The model under review builds one solid part; all positions refer to its coordinate system, in mm. A direction names the side the tool comes from. Round coordinates to 2 decimals unless told otherwise and drop trailing zeros.
1) Consider section A-A (z = 4.5). Give the number of separate pieces and of enclosed holes in the cut face, then the cut area to 3 significant figures.
2) Machinability: for faces 4 (the face through (11.156, 1.113, 11.154)), 5 (the face through (0, 5, 11)), which of the approach directions +Z, -Z, +X, -X, +Y, -Y give a long, thin tool a straight path to every point of the face, cutting with its end or side? Answer none if there is none.
3) Clearance check with flat-ended pins moving along their axes: P1, Ø2, axis at x = 8, z = 4, coming from the +Y side; P2, Ø5, axis at x = 14.5, z = 7.5, coming from the +Y side; P3, Ø3, axis at x = 12.5, z = 6, coming from the +Y side; P4, Ø6, axis at y = 3, z = 10, coming from the +X side. State where each tip first meets the part, or that it passes through.
4) To check wall thickness, follow L1, parallel to X at y = 2.75, z = 6; L2, parallel to Y at x = 6, z = 10.5; L3, parallel to X at y = 6.25, z = 20.5. State the ranges of each line that lie inside material, in increasing order.
5) Mouldability with a two-part tool opening along X and no side actions: class faces 1 (the face through (8, 5, 22)), 2 (the face through (19.386, 0.602, 11.154)), 3 (the face through (2.62, 5.38, 11.15)) as pulls with the +X half, pulls with the -X half, needs draft (parallel to the pull), parting line crosses it, or undercut.
from build123d import *

# Parameters (mm, degrees)
F0_R     = 1
F1_DEPTH = 22
F3_R     = 0.79999


# Not quite as in the source:
# - a fillet or chamfer is up to 0.001 mm smaller than in the source, because OpenCascade refuses the exact size
# - a feature of the source that left no trace in its solid (it failed there, or was rolled back) is left out


with BuildPart() as f1:
    # F0 (on Top) → F1 (new body)
    with BuildSketch(Plane.XY):
        Polygon((0, 10), (0, 0), (20, 0), (22, 0), (8.6841676623, 6.6579161689), (0, 11), align=None)
        with Locations((1.9193962216, 1.5117339551)):
            Circle(F0_R, mode=Mode.SUBTRACT)
        Polygon((3.0234679102, 6.6994116629), (9.2844582472, 3.5689164944), (11.9677398202, 2.2272757079), (11.6099689438, 1.5117339551), (11.2521980674, 0.7961922023), (9.8211145618, 1.5117339551), (7.0483902697, 2.8980961012), (4.3426890694, 4.2509467013), (2.3079261574, 5.2683281573), align=None, mode=Mode.SUBTRACT)
        with BuildLine():
            ThreePointArc((15.0937268734, 1.5117339551), (14.0937268734, 0.5117339551), (13.0937268734, 1.5117339551))
            ThreePointArc((13.0937268734, 1.5117339551), (14.0937268734, 2.5117339551), (15.0937268734, 1.5117339551))
        make_face(mode=Mode.SUBTRACT)
    extrude(amount=F1_DEPTH)

    # F3 (radius 0.8 in the source; OpenCascade refuses exactly that, so slightly less here)
    f3_edges = [f1.edges().sort_by_distance(p)[0] for p in [
        (0, 11, 11),
        (22, 0, 11),
        (11, 5.5, 0),
        (11, 5.5, 22),
        (0, 5.5, 22),
        (2.307926, 5.268328, 11),
        (3.023468, 6.699412, 11),
        (11.252198, 0.796192, 11),
        (11.96774, 2.227276, 11),
        (0, 0, 11),
        (0, 5.5, 0),
    ]]
    fillet(f3_edges, radius=F3_R)


solid = f1.part
Answer below:
1. separate pieces: 1
1. enclosed holes: 3
1. area: 96.9 mm2
2. face 4: +Z, -Z
2. face 5: +Z, -Z, -X, +Y, -Y
3. P1: stops at y = 7.5
3. P2: stops at y = 5
3. P3: stops at y = 5.5
3. P4: stops at x = 19.41
4. L1: x = 0 to 7.34, 10.92 to 16.5
4. L2: y = 0 to 3.42, 5.21 to 8
4. L3: x = 0 to 2.88, 3.92 to 9.5
5. face 1: needs draft
5. face 2: pulls with the +X half
5. face 3: undercut
